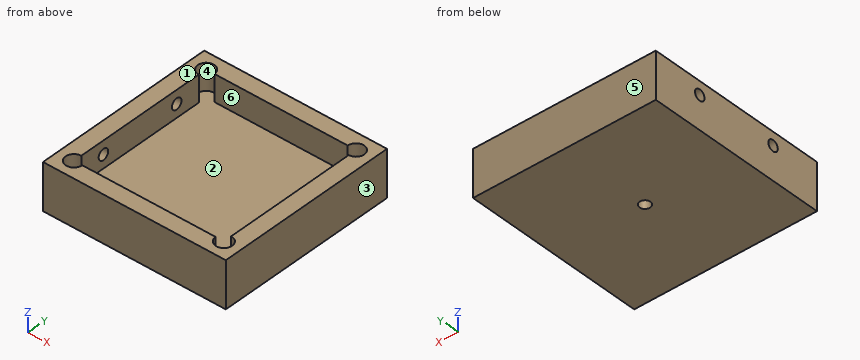
Autodesk Inventor part; units mm, degrees
ref_plane "YZ Plane" through (0, 0, 0) normal (1, 0, 0) x (0, 1, 0)
ref_plane "XZ Plane" through (0, 0, 0) normal (0, 1, 0) x (-1, 0, 0)
ref_plane "XY Plane" through (0, 0, 0) normal (0, 0, 1) x (1, 0, 0)
sketch "Sketch1" plane through (0, 0, 0) normal (0, 0, 1) x (1, 0, 0)
  line L0 (0, 38.5) -> (0, -38.5) construction
  line L1 (-38.5, 0) -> (38.5, 0) construction
  line L2 (-27.5, 27.5) -> (27.5, 27.5)
  line L3 (27.5, 27.5) -> (27.5, -27.5)
  line L4 (27.5, -27.5) -> (-27.5, -27.5)
  line L5 (-27.5, -27.5) -> (-27.5, 27.5)
  point P0 (0, 0)
  dimension "d0" = 55
  dimension "d1" = 55
extrude "Extrusion1" add sketch "Sketch1" along normal blind 20
sketch "Sketch4" plane through (0, 0, 20) normal (0, 0, 1) x (1, 0, 0)
  line L0 (-38.5, 0) -> (38.5, 0) construction
  line L1 (0, 38.5) -> (0, -38.5) construction
  line L2 (-22.55, 22.55) -> (22.55, 22.55) construction
  line L3 (22.55, 22.55) -> (22.55, -22.55) construction
  line L4 (22.55, -22.55) -> (-22.55, -22.55) construction
  line L5 (-22.55, -22.55) -> (-22.55, 22.55) construction
  point P0 (0, 0)
  dimension "d15" = 45.1
  dimension "d16" = 45.1
hole "Hole2" at (-22.55, 22.55, 20) at (22.55, 22.55, 20) at (22.55, -22.55, 20) at (-22.55, -22.55, 20) at (-22.55, 22.55, 20) at (22.55, 22.55, 20) direction (0, 0, -1) diameter 5 depth 8
sketch "Sketch5" plane through (0, 0, 20) normal (0, 0, 1) x (1, 0, 0)
  circle A0 centre (-22.55, 22.55) radius 2.5
  circle A1 centre (22.55, -22.55) radius 2.5
  line L0 (-22.55, 22.55) -> (22.55, 22.55)
  line L1 (22.55, 22.55) -> (22.55, -22.55)
  line L2 (22.55, -22.55) -> (-22.55, -22.55)
  line L3 (-22.55, -22.55) -> (-22.55, 22.55)
  point P0 (0, 0)
extrude "Extrusion3" cut sketch "Sketch5" against normal blind 8 contours L0 L1 A1 L2 L3 A0 | A0 L3 L0 | L1 L2 A1 picked at (-20.9042, 22.3646) picked at (22.003, -20.9868)
sketch "Sketch6" plane through (-27.5, -27.5, 0) normal (-1, 0, 0) x (0, 0, 1)
  line L0 (0, 55) -> (20, 55)
  line L1 (0, 0) -> (20, 0)
  line L2 (20, 7.45) -> (12, 7.45) construction
  line L3 (20, 47.55) -> (20, 7.45) construction
  line L4 (12, 47.55) -> (20, 47.55) construction
  line L5 (12, 7.45) -> (12, 47.55) construction
  line L6 (16, 47.55) -> (16, 7.45) construction
  point P0 (0, 27.5)
  point P1 (16, 40)
  point P2 (16, 15)
  dimension "d26" = 15
  dimension "d27" = 15
hole "Hole3" at (-27.5, 12.5, 16) at (-27.5, -12.5, 16) direction (1, 0, 0) diameter 3.242 end up to surface
sketch "Sketch8" plane through (0, 0, 0) normal (0, 0, -1) x (-1, 0, 0)
  line L0 (27.5, 27.5) -> (-27.5, 27.5) construction
  line L1 (-27.5, 27.5) -> (-27.5, -27.5) construction
  line L2 (-27.5, -27.5) -> (27.5, -27.5) construction
  line L3 (27.5, -27.5) -> (27.5, 27.5) construction
  line L4 (0, -38.5) -> (0, 38.5) construction
  line L5 (-38.5, 0) -> (38.5, 0) construction
  line L6 (-12.5, -12.5) -> (12.5, -12.5)
  line L7 (12.5, -12.5) -> (12.5, 12.5)
  line L8 (12.5, 12.5) -> (-12.5, 12.5)
  line L9 (-12.5, 12.5) -> (-12.5, -12.5)
  point P0 (0, 0)
  dimension "d44" = 25
  dimension "d45" = 25
extrude "Extrusion4" cut sketch "Sketch8" against normal blind 6
sketch "Sketch9" plane through (0, 0, 0) normal (0, 0, -1) x (-1, 0, 0)
  line L0 (12.5, 12.5) -> (12.5, -12.5) construction
  line L1 (12.5, -12.5) -> (-12.5, -12.5) construction
  line L2 (-12.5, -12.5) -> (-12.5, 12.5) construction
  line L3 (-12.5, 12.5) -> (12.5, 12.5) construction
  line L4 (27.5, 27.5) -> (-27.5, 27.5) construction
  line L5 (-27.5, 27.5) -> (-27.5, -27.5) construction
  line L6 (-27.5, -27.5) -> (27.5, -27.5) construction
  line L7 (27.5, -27.5) -> (27.5, 27.5) construction
  line L8 (12.5, -12.5) -> (-12.5, -12.5) construction
  point P0 (0, 0)
hole "Hole5" at (-12.5, 12.5, 0) at (-12.5, -12.5, 0) at (12.5, -12.5, 0) at (12.5, 12.5, 0) direction (0, 0, 1) diameter 3 depth 6
sketch "Sketch10" plane through (0, 0, 6) normal (0, 0, -1) x (-1, 0, 0)
  point P0 (0, 0)
  point P1 (0, 0)
hole "Hole6" at (0, 0, 6) direction (0, 0, 1) diameter 3.242 depth 4 tip angle 118
ref_plane "SplitPLane" through (0, 0, 6) normal (0, 0, -1) x (-1, 0, 0)
split "Split2" plane through (0, 0, 6) removes the side toward (0, 0, -1)
properties part number "Large-cuvette-mount-40mm-V4" material "PC/ABS Plastic"
Input: part model. Units: mm. Frame: model coordinates. Face numbers are marked on the shaded views. A direction names the side the tool comes from. Give positions to 0.01 mm unless a question says otherwise; leave off trailing zeros. Order: outer loops, then holes, each group sorted by start corner. A loop starts at its lowest first (then second) coordinate and runs counter-clockwise, first axis right, second up. Notation, with made-up numbers: (46.25, 62.25) - (78.25, 62.25) arc R25 cw to (78.25, 79.25) - close; hole circle Ø7 at (-38, 41.5). An arc over 180 degrees is marked (long way). Answer as a JSON object with one key per item and string values. Group by question number.
Q1. Cut plane A-A, the plane y = 12.5. Output: boundary loops of the cut face in (x, z), then the cut area to 3 significant figures.
Q2. Cut plane B-B, the plane y = -19. Output: boundary loops of the cut face in (x, z).
Q3. Line query: probe 1 along Z at (x, y) = (-24.7, -12.5); probe 2 along X at (y, z) = (0, 9.1); probe 3 along Y at (x, z) = (-3, 17.5). Output: solid intervals per line, ascending.
Q4. Cut plane C-C, the plane z = 15.25. Output: boundary loops of the cut face in (x, y), then the cut area to 3 significant figures.
Q5. Set-up query: the marked faces 1 and 2. Return all of +Z, -Z, +X, -X, +Y, -Y with unobstructed straight access to the full face (end or side cutting, diameter ignored); none if empty.
Q6. Mould query, pull axis X, two halves, no side actions, for the marked faces 3, 4, 5 and 6. Classes: pulls with the +X half, pulls with the -X half, needs draft (parallel to the pull), parting line crosses it, or undercut.
Q7. First-contact query: pin 1 Ø4 at (x, y) = (22.55, -22.55) entering from +Z; pin 2 Ø1.9 at (y, z) = (12.5, 16) entering from -X. Flat tips, straight axial feed; report the tip coordinate or a pass-through.
Q8. Cut plane D-D, the plane x = -23.5. Output: boundary loops of the cut face in (y, z).
Results:
{
 "1": {"outline": "(-27.5, 6) - (27.5, 6) - (27.5, 20) - (22.55, 20) - (22.55, 12) - (-22.55, 12) - (-22.55, 14.38) - (-27.5, 14.38) - close; (-27.5, 17.62) - (-22.55, 17.62) - (-22.55, 20) - (-27.5, 20) - close", "area": "393 mm^2"},
 "2": {"outline": "(-27.5, 6) - (27.5, 6) - (27.5, 20) - (22.55, 20) - (22.55, 12) - (-22.55, 12) - (-22.55, 20) - (-27.5, 20) - close"},
 "3": {"probe 1": "6 to 14.38, 17.62 to 20", "probe 2": "-27.5 to -1.62, 1.62 to 27.5", "probe 3": "-27.5 to -22.55, 22.55 to 27.5"},
 "4": {"outline": "(-27.5, -27.5) - (27.5, -27.5) - (27.5, 27.5) - (-27.5, 27.5) - (-27.5, 13.94) - (-22.55, 13.94) - (-22.55, 20.05) arc R2.5 cw (long way) to (-20.05, 22.55) - (20.05, 22.55) arc R2.5 cw (long way) to (22.55, 20.05) - (22.55, -20.05) arc R2.5 cw (long way) to (20.05, -22.55) - (-20.05, -22.55) arc R2.5 cw (long way) to (-22.55, -20.05) - (-22.55, -13.94) - (-27.5, -13.94) - close; (-27.5, -11.06) - (-22.55, -11.06) - (-22.55, 11.06) - (-27.5, 11.06) - close", "area": "904 mm^2"},
 "5": {"face 1": "+Z, +X, -X, +Y, -Y", "face 2": "+Z"},
 "6": {"face 3": "pulls with the +X half", "face 4": "undercut", "face 5": "needs draft", "face 6": "undercut"},
 "7": {"pin 1": "z = 12", "pin 2": "x = 22.55"},
 "8": {"outline": "(-27.5, 6) - (27.5, 6) - (27.5, 20) - (24.86, 20) - (24.86, 12) - (20.24, 12) - (20.24, 20) - (-20.24, 20) - (-20.24, 12) - (-24.86, 12) - (-24.86, 20) - (-27.5, 20) - close; hole circle Ø3.24 at (-12.5, 16); hole circle Ø3.24 at (12.5, 16)"}
}
